CAD build for the part. Positions are in the model's coordinates, mm. A direction names the side the tool comes from. Coordinates: 2 decimals unless noted, no trailing zeros. Loops run counter-clockwise (first coordinate to the right, second up) from the corner with the lowest first, then second, coordinate; pieces in that order, holes last. Notation, with made-up numbers: (-4, 64) -> (23, 64) arc R31 ccw to (23, 103) -> close; hole circle Ø5 at (61, 43.5). An arc over 180 degrees is marked (long way). Answer as a JSON object with one key per item and string values. Group by question number.
from build123d import *

# Parameters (mm, degrees)
SKETCH_W        = 200
SKETCH_H        = 250
PAD_DEPTH       = 15
SKETCH001_R     = 3.25
POCKET_DEPTH    = 15
SKETCH002_R     = 5.2
POCKET001_DEPTH = 6.2
SKETCH003_R     = 2.5
POCKET002_DEPTH = 15
SKETCH004_R     = 3.25
POCKET003_DEPTH = 15
SKETCH005_R     = 5.2
POCKET004_DEPTH = 7
SKETCH006_R     = 2.75
POCKET005_DEPTH = 15
SKETCH007_R     = 5
POCKET006_DEPTH = 6


with BuildPart() as part:
    # Sketch → Pad (new body)
    with BuildSketch(Plane.XY):
        with Locations((100, 125)):
            Rectangle(SKETCH_W, SKETCH_H)
    extrude(amount=PAD_DEPTH)

    # Sketch001 (on Face6 of Pad) → Pocket (cut)
    with BuildSketch(Plane.XY.offset(15)):
        with Locations((125, 37.5)):
            Circle(SKETCH001_R)
        with Locations((75, 37.5)):
            Circle(SKETCH001_R)
        with Locations((125, 112.5)):
            Circle(SKETCH001_R)
        with Locations((75, 112.5)):
            Circle(SKETCH001_R)
    extrude(amount=-POCKET_DEPTH, mode=Mode.SUBTRACT)

    # Sketch002 (on Face5 of Pocket) → Pocket001 (cut)
    with BuildSketch(Plane.XY.offset(15)):
        with Locations((75, 112.5)):
            Circle(SKETCH002_R)
        with Locations((125, 112.5)):
            Circle(SKETCH002_R)
        with Locations((75, 37.5)):
            Circle(SKETCH002_R)
        with Locations((125, 37.5)):
            Circle(SKETCH002_R)
    extrude(amount=-POCKET001_DEPTH, mode=Mode.SUBTRACT)

    # Sketch003 (on Face5 of Pocket001) → Pocket002 (cut)
    with BuildSketch(Plane.XY.offset(15)):
        with Locations((42, 230)):
            Circle(SKETCH003_R)
        with Locations((42, 125)):
            Circle(SKETCH003_R)
        with Locations((42, 20)):
            Circle(SKETCH003_R)
        with Locations((158, 230)):
            Circle(SKETCH003_R)
        with Locations((158, 125)):
            Circle(SKETCH003_R)
        with Locations((158, 20)):
            Circle(SKETCH003_R)
    extrude(amount=-POCKET002_DEPTH, mode=Mode.SUBTRACT)

    # Sketch004 (on Face5 of Pocket002) → Pocket003 (cut)
    with BuildSketch(Plane.XY.offset(15)):
        with Locations((40, 188.5)):
            Circle(SKETCH004_R)
        with Locations((80, 188.5)):
            Circle(SKETCH004_R)
        with Locations((120, 188.5)):
            Circle(SKETCH004_R)
        with Locations((160, 188.5)):
            Circle(SKETCH004_R)
    extrude(amount=-POCKET003_DEPTH, mode=Mode.SUBTRACT)

    # Sketch005 (on Face5 of Pocket003) → Pocket004 (cut)
    with BuildSketch(Plane.XY.offset(15)):
        with Locations((40, 188.5)):
            Circle(SKETCH005_R)
        with Locations((80, 188.5)):
            Circle(SKETCH005_R)
        with Locations((120, 188.5)):
            Circle(SKETCH005_R)
        with Locations((160, 188.5)):
            Circle(SKETCH005_R)
    extrude(amount=-POCKET004_DEPTH, mode=Mode.SUBTRACT)

    # Sketch006 (on Face5 of Pocket004) → Pocket005 (cut)
    with BuildSketch(Plane.XY.offset(15)):
        with Locations((26, 206)):
            Circle(SKETCH006_R)
        with Locations((58, 206)):
            Circle(SKETCH006_R)
        with Locations((26, 170)):
            Circle(SKETCH006_R)
        with Locations((58, 170)):
            Circle(SKETCH006_R)
        with Locations((26, 86)):
            Circle(SKETCH006_R)
        with Locations((58, 86)):
            Circle(SKETCH006_R)
        with Locations((26, 50)):
            Circle(SKETCH006_R)
        with Locations((58, 50)):
            Circle(SKETCH006_R)
        with Locations((142, 206)):
            Circle(SKETCH006_R)
        with Locations((174, 206)):
            Circle(SKETCH006_R)
        with Locations((142, 170)):
            Circle(SKETCH006_R)
        with Locations((174, 170)):
            Circle(SKETCH006_R)
        with Locations((142, 86)):
            Circle(SKETCH006_R)
        with Locations((174, 86)):
            Circle(SKETCH006_R)
        with Locations((142, 50)):
            Circle(SKETCH006_R)
        with Locations((174, 50)):
            Circle(SKETCH006_R)
    extrude(amount=-POCKET005_DEPTH, mode=Mode.SUBTRACT)

    # Sketch007 (on Face4 of Pocket005) → Pocket006 (cut)
    with BuildSketch(Plane(origin=(0, 0, 0), x_dir=(1, 0, 0), z_dir=(0, 0, -1))):
        with Locations((26, -50)):
            Circle(SKETCH007_R)
        with Locations((58, -50)):
            Circle(SKETCH007_R)
        with Locations((142, -50)):
            Circle(SKETCH007_R)
        with Locations((174, -50)):
            Circle(SKETCH007_R)
        with Locations((142, -86)):
            Circle(SKETCH007_R)
        with Locations((174, -86)):
            Circle(SKETCH007_R)
        with Locations((26, -86)):
            Circle(SKETCH007_R)
        with Locations((58, -86)):
            Circle(SKETCH007_R)
        with Locations((26, -170)):
            Circle(SKETCH007_R)
        with Locations((58, -170)):
            Circle(SKETCH007_R)
        with Locations((26, -206)):
            Circle(SKETCH007_R)
        with Locations((58, -206)):
            Circle(SKETCH007_R)
        with Locations((142, -170)):
            Circle(SKETCH007_R)
        with Locations((174, -170)):
            Circle(SKETCH007_R)
        with Locations((142, -206)):
            Circle(SKETCH007_R)
        with Locations((174, -206)):
            Circle(SKETCH007_R)
    extrude(amount=-POCKET006_DEPTH, mode=Mode.SUBTRACT)


solid = part.part
Item 1: Band-saw the part on B-B, the plane z = 2.5. Count the separate pieces of the cut face and the enclosed holes in it, and give its area (3 significant figures).
Item 2: Band-saw the part on A-A, the plane y = 37.5. List the corners of the cut face in (x, z), and give its area (3 significant figures).
Item 3: Drill centre lines: L1, parallel to X at y = 188.5, z = 4; L2, parallel to Y at x = 142, z = 12; L3, parallel to X at y = 206, z = 13.25. Where is each one in solid material? Low to high.
Item 4: Flat gauge pins, fed straight in: P1, Ø3, axis at x = 172, y = 171, coming from the -Z side; P2, Ø5, axis at x = 174, y = 170, coming from the +Z side; P3, Ø3, axis at x = 77.5, y = 39, coming from the +Z side; P4, Ø12, axis at x = 163, y = 125.5, coming from the -Z side. Where does each tip first touch, or does it go through?
Item 5: 3-axis set-ups, long thin cutter, end or side, ignore diameter. For faces 1 (the cylindrical face through (71.167, 41.014, 11.943)), 2 (the flat face through (28.2, 172.2, 6)), 3 (the cylindrical face through (55.818, 84.327, 10.563)): which of +Z, -Z, +X, -X, +Y, -Y reach the whole face in a straight line?
Reply:
{
 "1": {"separate pieces": "1", "enclosed holes": "30", "area": "48,400 mm²"},
 "2": {"outline": "(0, 0) -> (71.75, 0) -> (71.75, 8.8) -> (69.8, 8.8) -> (69.8, 15) -> (0, 15) -> close; (78.25, 0) -> (121.75, 0) -> (121.75, 8.8) -> (119.8, 8.8) -> (119.8, 15) -> (80.2, 15) -> (80.2, 8.8) -> (78.25, 8.8) -> close; (128.25, 0) -> (200, 0) -> (200, 15) -> (130.2, 15) -> (130.2, 8.8) -> (128.25, 8.8) -> close", "area": "2,760 mm²"},
 "3": {"L1": "0 to 36.75, 43.25 to 76.75, 83.25 to 116.75, 123.25 to 156.75, 163.25 to 200", "L2": "0 to 47.25, 52.75 to 83.25, 88.75 to 167.25, 172.75 to 203.25, 208.75 to 250", "L3": "0 to 23.25, 28.75 to 55.25, 60.75 to 139.25, 144.75 to 171.25, 176.75 to 200"},
 "4": {"P1": "z = 6", "P2": "through", "P3": "z = 8.8", "P4": "z = 0"},
 "5": {"face 1": "+Z", "face 2": "-Z", "face 3": "+Z, -Z"}
}
